from build123d import *

# Parameters (mm, degrees)
SKETCH_1_R          = 3.175
EXTRUDE_1_DEPTH     = 57.15
CUT_EXTRUDE_1_DEPTH = 10.795
SKETCH_3_R          = 0.889
CUT_EXTRUDE_2_DEPTH = 10.795
SKETCH_4_W          = 3.926157487
SKETCH_4_H          = 0.79375
CUT_EXTRUDE_3_DEPTH = 8.573


with BuildPart() as part:
    # 草图1 → 凸台-拉伸1 (new body)
    with BuildSketch(Plane(origin=(0, 0, 0), x_dir=(1, 0, 0), z_dir=(0, 1, 0))):
        Circle(SKETCH_1_R)
    extrude(amount=EXTRUDE_1_DEPTH)

    # 草图2 → 切除-拉伸1 (cut)
    with BuildSketch(Plane(origin=(0, 57.15, 0), x_dir=(1, 0, 0), z_dir=(0, 1, 0))):
        Polygon((-0.794, 3.175), (0.794, 3.175), (0.794, -3.175), (-3.175, -3.175), (-3.175, 3.175), align=None)
    extrude(amount=-CUT_EXTRUDE_1_DEPTH, mode=Mode.SUBTRACT)

    # 草图3 → 切除-拉伸2 (cut)
    with BuildSketch(Plane.ZY.offset(-0.794)):
        with Locations((0, 53.855)):
            Circle(SKETCH_3_R)
        with Locations((0, 48.855)):
            Circle(SKETCH_3_R)
    extrude(amount=-CUT_EXTRUDE_2_DEPTH, mode=Mode.SUBTRACT)

    # 草图4 → 切除-拉伸3 (cut)
    with BuildSketch(Plane.XZ):
        with Locations((-0.018009896, -2.778125)):
            Rectangle(SKETCH_4_W, SKETCH_4_H)
    extrude(amount=-CUT_EXTRUDE_3_DEPTH, mode=Mode.SUBTRACT)


solid = part.part
For this review, take the finished solid that the model builds, in its own axes (mm). A direction names the side the tool comes from. Give positions to 0.01 mm unless a question says otherwise; leave off trailing zeros. Loops run counter-clockwise (first coordinate to the right, second up) from the corner with the lowest first, then second, coordinate; pieces in that order, holes last. Notation, with made-up numbers: (87, -23.5) -> (143, -23.5) arc R12 cw to (143, -13.5) -> close; hole circle Ø10 at (40.25, 49.25). An arc over 180 degrees is marked (long way). One line per question, with ' | ' between items.
1) We need section A-A (z = 0). Write out the cut boundary in (x, y) (3 decimals).
Resolved:
outline: (-3.175, 0) -> (3.175, 0) -> (3.175, 47.966) -> (0.794, 47.966) -> (0.794, 46.355) -> (-3.175, 46.355) -> close; (0.794, 49.744) -> (3.175, 49.744) -> (3.175, 52.966) -> (0.794, 52.966) -> close; (0.794, 54.744) -> (3.175, 54.744) -> (3.175, 57.15) -> (0.794, 57.15) -> close
2) Insertion check: pin 1 Ø1 at (x, y) = (-2.5, 20) entering from -Z; pin 2 Ø1 at (y, z) = (42, 1.5) entering from -X; pin 3 Ø2 at (y, z) = (24, -2) entering from +X; pin 4 Ø3 at (y, z) = (53.855, 0) entering from +X (3 decimals). Each pin has a flat end and moves straight along its axis. Give the tip position at first contact, or say it passes through.
Resolved:
pin 1: stops at z = -2.47 | pin 2: stops at x = -3.01 | pin 3: stops at x = 3.01 | pin 4: stops at x = 3.175
3) We need section D-D (z = 2.25). Write out the cut boundary in (x, y) (3 decimals).
Resolved:
outline: (-2.24, 0) -> (2.24, 0) -> (2.24, 57.15) -> (0.794, 57.15) -> (0.794, 46.355) -> (-2.24, 46.355) -> close
4) We need section B-B (y = 14). Write out the cut boundary in (x, z) (3 decimals), plus the area to 3 significant figures.
Resolved:
outline: circle Ø6.35 at (0, 0) | area: 31.7 mm2
5) For faces 5 (the flat face through (-1, 46.355, 0)), 6 (the flat face through (0, 0, 0)), list the 3-axis set-ups (+Z, -Z, +X, -X, +Y, -Y) from which the entire face can be reached by the end or side of a thin tool; tool diameter is ignored.
Resolved:
face 5: +Z, -Z, -X, +Y | face 6: +Z, -Z, +X, -X, -Y
6) We need section C-C (x = 0). Write out the cut boundary in (y, z) (3 decimals), plus the area to 3 significant figures.
Resolved:
outline: (0, -2.381) -> (8.573, -2.381) -> (8.573, -3.175) -> (46.355, -3.175) -> (46.355, 3.175) -> (0, 3.175) -> close | area: 288 mm2
7) To check wall thickness, follow probe 1 along Y at (x, z) = (1.9, 0); probe 2 along Y at (x, z) = (-1.5, 0.25) (3 decimals); probe 3 along X at (y, z) = (20.5, 1.5). State the ranges of each line that lie inside material, in increasing order.
Resolved:
probe 1: y = 0 to 47.97, 49.74 to 52.97, 54.74 to 57.15 | probe 2: y = 0 to 46.355 | probe 3: x = -2.8 to 2.8
8) The part is to be moulded in two halves that separate along Z. For faces 1 (the cylindrical face through (1.968, 52.987, -0.193)), 2 (the flat face through (0, 4, -2.381)), 3 (the cylindrical face through (1.968, 47.987, -0.193)), 4 (the flat face through (2, 57.15, 0)), say which applies: +Z half, -Z half, draft (parallel to the pull), parting line (faces both ways), or undercut.
Resolved:
face 1: undercut | face 2: -Z half | face 3: undercut | face 4: draft
